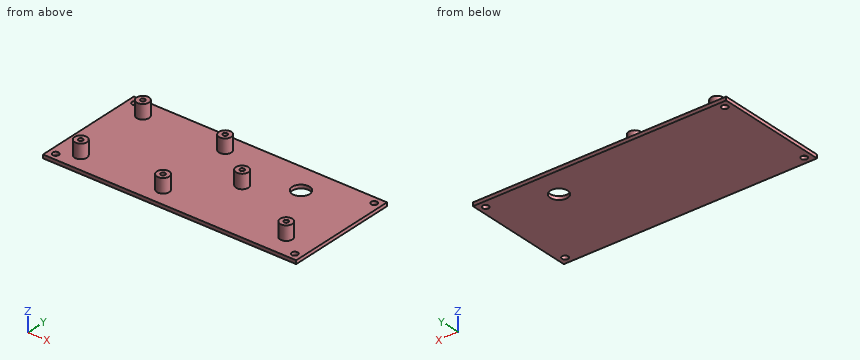
from build123d import *

# Parameters (mm, degrees)
F0_R     = 1.397
F0_R_2   = 2.794
F0_R_3   = 3.937
F0_R_4   = 1.016
F1_DEPTH = 1.5875
F2_DEPTH = 6.35


with BuildPart() as f1:
    # F0 (on Top) → F1 (new body)
    with BuildSketch(Plane.XY):
        Polygon((53.848, -25.273), (57.023, -25.273), (57.023, -22.098), (57.023, 22.098), (57.023, 25.273), (53.848, 25.273), (-53.848, 25.273), (-57.023, 25.273), (-57.023, 22.098), (-57.023, -22.098), (-57.023, -25.273), (-53.848, -25.273), align=None)
        with Locations((-53.848, -22.098)):
            Circle(F0_R, mode=Mode.SUBTRACT)
        with Locations((-46.482, -17.272)):
            Circle(F0_R_2, mode=Mode.SUBTRACT)
        with Locations((-9.398, -17.272)):
            Circle(F0_R_2, mode=Mode.SUBTRACT)
        with Locations((53.848, -22.098)):
            Circle(F0_R, mode=Mode.SUBTRACT)
        with Locations((44.323, -15.113)):
            Circle(F0_R_2, mode=Mode.SUBTRACT)
        with Locations((-46.482, 17.272)):
            Circle(F0_R_2, mode=Mode.SUBTRACT)
        with Locations((-53.848, 22.098)):
            Circle(F0_R, mode=Mode.SUBTRACT)
        with Locations((-9.398, 17.272)):
            Circle(F0_R_2, mode=Mode.SUBTRACT)
        with Locations((10.287, 2.413)):
            Circle(F0_R_2, mode=Mode.SUBTRACT)
        with Locations((28.5115, 12.6365)):
            Circle(F0_R_3, mode=Mode.SUBTRACT)
        with Locations((53.848, 22.098)):
            Circle(F0_R, mode=Mode.SUBTRACT)
        with Locations((-9.398, 17.272)):
            Circle(F0_R_2)
        with Locations((-9.398, 17.272)):
            Circle(F0_R_4, mode=Mode.SUBTRACT)
        with Locations((-9.398, -17.272)):
            Circle(F0_R_2)
        with Locations((-9.398, -17.272)):
            Circle(F0_R_4, mode=Mode.SUBTRACT)
        with Locations((-46.482, -17.272)):
            Circle(F0_R_2)
        with Locations((-46.482, -17.272)):
            Circle(F0_R_4, mode=Mode.SUBTRACT)
        with Locations((-46.482, 17.272)):
            Circle(F0_R_2)
        with Locations((-46.482, 17.272)):
            Circle(F0_R_4, mode=Mode.SUBTRACT)
        with Locations((10.287, 2.413)):
            Circle(F0_R_2)
        with Locations((10.287, 2.413)):
            Circle(F0_R_4, mode=Mode.SUBTRACT)
        with Locations((44.323, -15.113)):
            Circle(F0_R_2)
        with Locations((44.323, -15.113)):
            Circle(F0_R_4, mode=Mode.SUBTRACT)
        with Locations((-9.398, 17.272)):
            Circle(F0_R_4)
        with Locations((-9.398, -17.272)):
            Circle(F0_R_4)
        with Locations((-46.482, -17.272)):
            Circle(F0_R_4)
        with Locations((-46.482, 17.272)):
            Circle(F0_R_4)
        with Locations((10.287, 2.413)):
            Circle(F0_R_4)
        with Locations((44.323, -15.113)):
            Circle(F0_R_4)
    extrude(amount=-F1_DEPTH)

    # F0 (on Top) → F2 (join)
    with BuildSketch(Plane.XY):
        with Locations((10.287, 2.413)):
            Circle(F0_R_2)
        with Locations((10.287, 2.413)):
            Circle(F0_R_4, mode=Mode.SUBTRACT)
        with Locations((44.323, -15.113)):
            Circle(F0_R_2)
        with Locations((44.323, -15.113)):
            Circle(F0_R_4, mode=Mode.SUBTRACT)
        with Locations((-9.398, -17.272)):
            Circle(F0_R_2)
        with Locations((-9.398, -17.272)):
            Circle(F0_R_4, mode=Mode.SUBTRACT)
        with Locations((-9.398, 17.272)):
            Circle(F0_R_2)
        with Locations((-9.398, 17.272)):
            Circle(F0_R_4, mode=Mode.SUBTRACT)
        with Locations((-46.482, 17.272)):
            Circle(F0_R_2)
        with Locations((-46.482, 17.272)):
            Circle(F0_R_4, mode=Mode.SUBTRACT)
        with Locations((-46.482, -17.272)):
            Circle(F0_R_2)
        with Locations((-46.482, -17.272)):
            Circle(F0_R_4, mode=Mode.SUBTRACT)
    extrude(amount=F2_DEPTH)


solid = f1.part
Read the model definition and answer for the solid it produces. Units are mm, in the model's axes. Give positions to 0.01 mm unless a question says otherwise; leave off trailing zeros. Loops run counter-clockwise (first coordinate to the right, second up) from the corner with the lowest first, then second, coordinate; pieces in that order, holes last. Notation, with made-up numbers: (-36, 1) -> (-16, 1) arc R26 cw to (-16, 16) -> close; hole circle Ø10 at (-37, 18). An arc over 180 degrees is marked (long way). Answer as CSV lines item,"result".
Item 1: Find section B-B on x = 29. Give the vertices of the cut face in (y, z).
Returned:
outline,"(-25.27, -1.59) -> (8.73, -1.59) -> (8.73, 0) -> (-25.27, 0) -> close; (16.54, -1.59) -> (25.27, -1.59) -> (25.27, 0) -> (16.54, 0) -> close"
Item 2: Find section A-A on z = 5. State how many separate pieces and enclosed holes the cut face has, plus the area to 3 significant figures.
Returned:
separate pieces,"6"
enclosed holes,"6"
area,"128 mm²"
Item 3: Consider line 1 (X direction, y = -17.5, z = 1.5); line 2 (Z direction, x = 13.5, y = -20); line 3 (X direction, y = 9.5, z = -1). Determine where each line is inside the solid, lowest interval first. Write a range as [from, to].
Returned:
line 1,"x = [-49.27, -47.47], [-45.49, -43.7], [-12.18, -10.39], [-8.41, -6.61], [42.87, 45.78]"
line 2,"z = [-1.59, 0]"
line 3,"x = [-57.02, 26.13], [30.89, 57.02]"
Item 4: Find section C-C on y = -6.5. Give the vertices of the cut face in (x, z).
Returned:
outline,"(-57.02, -1.59) -> (57.02, -1.59) -> (57.02, 0) -> (-57.02, 0) -> close"
Item 5: Each of these flat-tipped pins is pushed along its axis until it touches: pin 1 (2 mm diameter, centred on x = -9, y = 17, fed in from +Z); pin 2 (5 mm diameter, centred on x = 2, y = -12, fed in from +Z). Where does it stop, or does it pass through?
Returned:
pin 1,"stops at z = 6.35"
pin 2,"stops at z = 0"
